Input: part model. Units: mm. Frame: model coordinates. A direction names the side the tool comes from. Coordinates: 2 decimals unless noted, no trailing zeros. Write each loop counter-clockwise with the first axis right and the second up, starting at its lowest first coordinate (ties: lowest second). Pieces come first, ordered by that corner, then holes.
from build123d import *

# Parameters (mm, degrees)
ESBO_O1_R                = 4
RESSALTO_EXTRUS_O2_DEPTH = 10
ESBO_O2_W                = 80
ESBO_O2_H                = 124.892668507
ESBO_O2_R                = 2.5
RESSALTO_EXTRUS_O3_DEPTH = 5
FILETE5_R                = 2
FILETE6_R                = 5
FILETE7_R                = 10
CHANFRO1_SIZE            = 1


with BuildPart() as part:
    # Esbo_o1 → Ressalto-extrus_o2 (new body)
    with BuildSketch(Plane(origin=(10, 0, 0), x_dir=(0, 0, -1), z_dir=(1, 0, 0))):
        with BuildLine():
            Line((51.839732536, -73.052935971), (0, -124.892668507))
            Line((0, -124.892668507), (0, 0))
            Line((0, 0), (51.839732536, -51.839732536))
            ThreePointArc((51.839732536, -51.839732536), (56.233130818, -62.446334254), (51.839732536, -73.052935971))
        make_face()
        with Locations((41.233130818, -62.446334254)):
            Circle(ESBO_O1_R, mode=Mode.SUBTRACT)
        Polygon((10, -24.142135624), (10, -58.553710058), (27.205787217, -41.347922841), align=None, mode=Mode.SUBTRACT)
        Polygon((10, -100.750532883), (27.205787217, -83.544745666), (10, -66.338958449), align=None, mode=Mode.SUBTRACT)
        Polygon((27.205787217, -48.418990653), (27.205787217, -76.473677854), (13.178443616, -62.446334254), align=None, mode=Mode.SUBTRACT)
    extrude(amount=RESSALTO_EXTRUS_O2_DEPTH)


with BuildPart() as body_2:
    # Espelhar2: mirrored copy
    add(part.part.mirror(Plane(origin=(0, 0, 0), x_dir=(0, 0, 1), z_dir=(1, 0, 0))))


with BuildPart() as part_1:
    add(part.part)

    add(body_2.part)  # Ressalto-extrus_o3 merges body 2
    # Esbo_o2 → Ressalto-extrus_o3 (add)
    with BuildSketch(Plane.XY):
        with Locations((0, -62.446334254)):
            Rectangle(ESBO_O2_W, ESBO_O2_H)
        with Locations((-30, -10)):
            Circle(ESBO_O2_R, mode=Mode.SUBTRACT)
        with Locations((30, -10)):
            Circle(ESBO_O2_R, mode=Mode.SUBTRACT)
        with Locations((-30, -114.892668507)):
            Circle(ESBO_O2_R, mode=Mode.SUBTRACT)
        with Locations((30, -114.892668507)):
            Circle(ESBO_O2_R, mode=Mode.SUBTRACT)
        with Locations((0, -114.892668507)):
            Circle(ESBO_O2_R, mode=Mode.SUBTRACT)
    extrude(amount=RESSALTO_EXTRUS_O3_DEPTH)

    # Filete5
    filete5_edges = [part_1.edges().sort_by_distance(p)[0] for p in [
        (15, -100.750532883, -10),
        (15, -83.544745666, -27.205787217),
        (15, -66.338958449, -10),
        (15, -24.142135624, -10),
        (15, -58.553710058, -10),
        (15, -41.347922841, -27.205787217),
        (15, -76.473677854, -27.205787217),
        (15, -48.418990653, -27.205787217),
        (15, -62.446334254, -13.178443616),
    ]]
    fillet(filete5_edges, radius=FILETE5_R)

    # Filete6
    filete6_edges = [part_1.edges().sort_by_distance(p)[0] for p in [
        (10, -62.446334254, 0),
        (20, -62.446334254, 0),
        (-10, -62.446334254, 0),
        (-20, -62.446334254, 0),
    ]]
    fillet(filete6_edges, radius=FILETE6_R)

    # Filete7
    filete7_edges = [part_1.edges().sort_by_distance(p)[0] for p in [
        (-40, 0, 2.5),
        (-40, -124.892668507, 2.5),
        (40, -124.892668507, 2.5),
        (40, 0, 2.5),
    ]]
    fillet(filete7_edges, radius=FILETE7_R)

    # Chanfro1
    chanfro1_edges = [part_1.edges().sort_by_distance(p)[0] for p in [
        (0, -124.892668507, 5),
        (-40, -62.446334254, 5),
        (40, -62.446334254, 5),
        (0, 0, 5),
        (37.071067812, -2.928932188, 5),
        (-37.071067812, -2.928932188, 5),
        (37.071067812, -121.963736319, 5),
        (-37.071067812, -121.963736319, 5),
        (-32.5, -10, 5),
        (27.5, -10, 5),
        (-32.5, -114.892668507, 5),
        (27.5, -114.892668507, 5),
        (-2.5, -114.892668507, 5),
    ]]
    chamfer(chanfro1_edges, length=CHANFRO1_SIZE)


solid = part_1.part
Item 1: Pin query (flat end, axial travel): pin 1 Ø6.5 at (x, y) = (-30, -10) entering from +Z; pin 2 Ø8 at (x, y) = (30, -114.89) entering from -Z; pin 3 Ø15.5 at (y, z) = (-56, -22.5) entering from -X. Return the tip coordinate at first contact, or that it passes through.
Item 2: Section query D-D, the plane z = -22. State how many separate pieces and enclosed holes the cut face has, then the cut area to 3 significant figures.
Item 3: Section query B-B, the plane z = -28.5. Return loops of the section in (x, y), then the cut area to 3 significant figures.
Item 4: Section query A-A, the plane x = 0. Return loops of the section in (y, z), then the cut area to 3 significant figures.
Item 5: Access query for faces 4 (the face through (-14.93, -75.06, -18.72)), 5 (the face through (15, -41, -10)), 6 (the face through (-33, -62, 0)), 7 (the face through (29.46, -12.44, 1.97)). Directions: +Z, -Z, +X, -X, +Y, -Y. A direction counts if a zero-diameter tool reaches every point of the face in a straight line with its end or side. Return the directions, or none.
Item 6: Pull-direction query (Z, two-part tool) for faces 1 (the face through (15.07, -51.41, -26)), 2 (the face through (20, -62, -31)), 3 (the face through (36.41, -121.44, 4.84)); classes: released by +Z, released by -Z, zero draft, split by the parting line, or undercut.
Item 7: Material intervals for line 1 (Y direction, x = 30, z = 2.25); line 2 (X direction, y = -66, z = -13); line 3 (Y direction, x = 0, z = 2.95), sorted ascending.
Item 8: Section query C-C, the plane x = -17. Return loops of the section in (y, z).
The answers:
1. pin 1: stops at z = 4.75
1. pin 2: stops at z = 0
1. pin 3: stops at x = -20
2. separate pieces: 8
2. enclosed holes: 0
2. area: 849 mm2
3. outline: (-20, -96.39) - (-10, -96.39) - (-10, -28.5) - (-20, -28.5) - close; (10, -96.39) - (20, -96.39) - (20, -28.5) - (10, -28.5) - close
3. area: 1,360 mm2
4. outline: (-124.89, 0) - (-117.39, 0) - (-117.39, 4) - (-118.39, 5) - (-123.89, 5) - (-124.89, 4) - close; (-112.39, 0) - (0, 0) - (0, 4) - (-1, 5) - (-111.39, 5) - (-112.39, 4) - close
4. area: 597 mm2
5. face 4: -X
5. face 5: +X, -X
5. face 6: -Z, -X, +Y, -Y
5. face 7: +Z, -Z
6. face 1: undercut
6. face 2: zero draft
6. face 3: released by +Z
7. line 1: y = -124.89 to -117.39, -112.39 to -12.5, -7.5 to 0
7. line 2: x = -20 to -10, 10 to 20
7. line 3: y = -124.89 to -117.39, -112.39 to 0
8. outline: (-124.89, 0) - (-73.05, -51.84) arc R15 ccw to (-51.84, -51.84) - (0, 0) - (0, 4) - (-1, 5) - (-123.89, 5) - (-124.89, 4) - close; hole (-100.75, -10) - (-83.54, -27.21) - (-66.34, -10) - close; hole (-76.47, -27.21) - (-48.42, -27.21) - (-62.45, -13.18) - close; hole circle Ø8 at (-62.45, -41.23); hole (-58.55, -10) - (-41.35, -27.21) - (-24.14, -10) - close
